```python
from build123d import *

# Parameters (mm, degrees)
ESQUISSE1_W             = 21
ESQUISSE1_H             = 21
BOSS_EXTRU_1_DEPTH      = 50
ESQUISSE3_W             = 21
ESQUISSE3_H             = 21
BOSS_EXTRU_2_DEPTH      = 30
COQUE1_T                = -0.5
CONG_1_R                = 2
ESQUISSE4_R             = 1.5
ENL_V_MAT_EXTRU_1_DEPTH = 68.684931853


with BuildPart() as part:
    # Esquisse1 → Boss.-Extru.1 (new body)
    with BuildSketch(Plane.XY):
        Rectangle(ESQUISSE1_W, ESQUISSE1_H)
    extrude(amount=BOSS_EXTRU_1_DEPTH)

    # Esquisse3 → Boss.-Extru.2 (add)
    with BuildSketch(Plane.XZ.offset(10.5)):
        with Locations((0, 10.5)):
            Rectangle(ESQUISSE3_W, ESQUISSE3_H)
    extrude(amount=BOSS_EXTRU_2_DEPTH)

    # Coque1
    coque1_openings = [part.faces().sort_by_distance(p)[0] for p in [
        (0, 0, 50),
        (0, -40.5, 10.5),
    ]]
    offset(amount=COQUE1_T, openings=coque1_openings, kind=Kind.INTERSECTION)

    # Congé1
    cong_1_edges = [part.edges().sort_by_distance(p)[0] for p in [
        (0, 10.5, 0),
    ]]
    fillet(cong_1_edges, radius=CONG_1_R)

    # Esquisse4 → Enlèv. mat.-Extru.1 (cut, through all)
    with BuildSketch(Plane.ZY.offset(10.5)):
        with Locations(Location((8, -6.690777593, 0), (0, 0, 270))):
            Circle(ESQUISSE4_R)
    extrude(amount=-ENL_V_MAT_EXTRU_1_DEPTH, mode=Mode.SUBTRACT)


solid = part.part
```
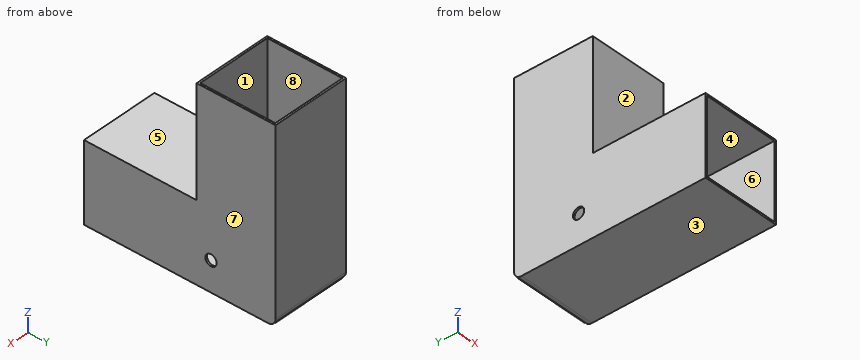
Read the model definition and answer for the solid it produces. Units are mm, in the model's axes. Face numbers are marked on the shaded views. A direction names the side the tool comes from. Give positions to 0.01 mm unless a question says otherwise; leave off trailing zeros. Write each loop counter-clockwise with the first axis right and the second up, starting at its lowest first coordinate (ties: lowest second). Pieces come first, ordered by that corner, then holes. Notation, with made-up numbers: (72, 25.5) - (113, 25.5) arc R21 cw to (113, 49.5) - close; hole circle Ø2 at (-20.5, 67). An arc over 180 degrees is marked (long way). Write item = value, one per line. Start each with the question number.
Item 1: A tool of negligible diameter and unlimited length cuts with its end or side. For the marked faces 1, 2, 3 and 4, from which of +Z, -Z, +X, -X, +Y, -Y can it reach the whole face along a straight path? Write none if from no direction.
Item 2: Find the intervals of material crossed by probe 1 along Y at (x, z) = (7.75, 23.5); probe 2 along Z at (x, y) = (-4.25, -24.5), in increasing order. Write a range as [from, to].
Item 3: Find section D-D (z = 27.5). Give the vertices of the cut face in (x, y), then the cut area to 3 significant figures.
Item 4: Each of these flat-tipped pins is pushed along its axis until it touches: P1, Ø5, axis at x = -7, z = 27.5, coming from the -Y side; P2, Ø8, axis at x = 3.5, z = 16, coming from the -Y side; P3, Ø3.5, axis at y = -6.69, z = 8, coming from the -X side; P4, Ø10, axis at x = 3, y = -17, coming from the +Z side. Where does it stop, or does it pass through?
Item 5: The mould has two halves that part along X. Classify the marked faces 5, 6, 7 and 8: +X half, -X half, draft (parallel to the pull), parting line (faces both ways), or undercut.
Item 6: Find section A-A (z = 8). Give the vertices of the cut face in (x, y).
Item 7: Find section B-B (y = -1.5). Give the vertices of the cut face in (x, z).
Response:
q1.face_1 = +Z
q1.face_2 = +Z, +X, -X, -Y
q1.face_3 = -Z, +X, -X, +Y, -Y
q1.face_4 = -Y
q2.probe_1 = [-10.5, -10], [10, 10.5]
q2.probe_2 = [0, 0.5], [20.5, 21]
q3.outline = (-10.5, -10.5) - (10.5, -10.5) - (10.5, 10.5) - (-10.5, 10.5) - close; hole (-10, -10) - (10, -10) - (10, 10) - (-10, 10) - close
q3.area = 41.0 mm²
q4.P1 = -10.5
q4.P2 = 10
q4.P3 = -10.5
q4.P4 = 21
q5.face_5 = draft
q5.face_6 = undercut
q5.face_7 = +X half
q5.face_8 = undercut
q6.outline = (-10.5, -40.5) - (-10, -40.5) - (-10, -8.19) - (-10.5, -8.19) - close; (-10.5, -5.19) - (-10, -5.19) - (-10, 10) - (10, 10) - (10, -5.19) - (10.5, -5.19) - (10.5, 10.5) - (-10.5, 10.5) - close; (10, -40.5) - (10.5, -40.5) - (10.5, -8.19) - (10, -8.19) - close
q7.outline = (-10.5, 0) - (10.5, 0) - (10.5, 50) - (10, 50) - (10, 0.5) - (-10, 0.5) - (-10, 50) - (-10.5, 50) - close
